Autodesk Inventor part; units mm, degrees
ref_plane "YZ Plane" through (0, 0, 0) normal (1, 0, 0) x (0, 1, 0)
ref_plane "XZ Plane" through (0, 0, 0) normal (0, 1, 0) x (-1, 0, 0)
ref_plane "XY Plane" through (0, 0, 0) normal (0, 0, 1) x (1, 0, 0)
sketch "草圖1" plane through (0, 0, 0) normal (0, 0, 1) x (1, 0, 0)
  line L0 (0, 0) -> (0, -20)
  line L1 (0, -20) -> (-115, -20)
  line L2 (0, -20) -> (450, -20)
  line L3 (167.5, 0) -> (430, 0)
  line L4 (167.5, 0) -> (-95, 0)
  line L5 (167.5, 75) -> (470, 75)
  line L6 (470, 75) -> (430, 0)
  line L7 (167.5, 75) -> (-135, 75)
  line L8 (-135, 75) -> (-95, 0)
  line L9 (130, 0) -> (130, 75)
  line L10 (130, 0) -> (150, 0)
  line L11 (150, 0) -> (150, 75)
  line L12 (167.5, 95) -> (545, 95)
  line L13 (545, 95) -> (545, 75)
  line L14 (545, 75) -> (500, 75)
  line L15 (500, 75) -> (450, -20)
  line L16 (-115, -20) -> (-165.6667, 75)
  line L17 (-165.6667, 75) -> (-210.6667, 75)
  line L18 (-210.6667, 75) -> (-210.6667, 95)
  line L19 (-210.6667, 95) -> (167.5, 95)
  dimension "d0" = 20
  dimension "d1" = 115
  dimension "d2" = 450
  dimension "d6" = 262.5
  dimension "d7" = 262.5
  dimension "d8" = 302.5
  dimension "d9" = 302.5
  dimension "d11" = 20
  dimension "d12" = 75
  dimension "d14" = 377.5
  dimension "d15" = 20
  dimension "d16" = 45
  dimension "d17" = 45
  dimension "d18" = 20
extrude "擠出1" add sketch "草圖1" along normal blind 20 contours L1 L16 L17 L18 L19 L12 L13 L14 L15 L2 | L9 L7 L11 L4
sketch "草圖2" plane through (-210.6667, 95, 0) normal (0, 1, 0) x (1, 0, 0)
  line L0 (0, 0) -> (0, -20)
  circle A0 centre (0, -10) radius 32.5
  circle A1 centre (32.5, -10) radius 5
  line L1 (755.6667, 0) -> (755.6667, -20)
  circle A2 centre (755.6667, -10) radius 32.5
  circle A3 centre (723.1667, -10) radius 5
  point P0 (210.6667, 0)
  dimension "d21" = 65
  dimension "d23" = 65
  dimension "d22" = 10
  dimension "d24" = 10
extrude "擠出2" add sketch "草圖2" along normal blind 20 contours A0 A1 | A0 A1 | A3 A2 | A2 A3 picked at (30.8705, -10.9665) picked at (33.9711, -11.3119) picked at (724.8619, -10) picked at (721.5286, -10)
sketch "草圖3" plane through (512.5, 115, 10) normal (0, 1, 0) x (1, 0, 0)
  circle A0 centre (0, 0) radius 17.5
  point P0 (-512.5, 10)
  dimension "d27" = 35
extrude "擠出3" add sketch "草圖3" along normal blind 10
sketch "草圖4" plane through (-178.1667, 115, 10) normal (0, 1, 0) x (1, 0, 0)
  circle A0 centre (0, 0) radius 5
  circle A1 centre (0, 0) radius 17.5
  point P0 (178.1667, 10)
  dimension "d30" = 35
extrude "擠出4" add sketch "草圖4" along normal blind 10 contours A0 | A1
properties part number "DOF8"
Geometry: final body of the model. Coordinates: model frame, mm. A direction names the side the tool comes from. Round coordinates to 2 decimals unless told otherwise and drop trailing zeros. Write each loop counter-clockwise with the first axis right and the second up, starting at its lowest first coordinate (ties: lowest second). Pieces come first, ordered by that corner, then holes. Notation, with made-up numbers: (21.5, 77) -> (34.5, 77) arc R19 cw to (34.5, 109) -> close; hole circle Ø3 at (67, 0.25). An arc over 180 degrees is marked (long way). Return JSON: item names as keys, results as strings.
Q1. Mould query, pull axis Y, two halves, no side actions, for faces 5 (the flat face through (-210.667, 85, 10)), 6 (the flat face through (-188, 75, 10)), 7 (the flat face through (512, 125, 10)), 8 (the flat face through (516, 115, 14)). Classes: +Y half, -Y half, draft (parallel to the pull), parting line (faces both ways), or undercut.
From the geometry:
{"face 5": "draft", "face 6": "-Y half", "face 7": "+Y half", "face 8": "undercut"}
Q2. Section C-C on y = -8.5. Return the cut outline in (x, z).
From the geometry:
{"outline": "(-121.13, 0) -> (456.05, 0) -> (456.05, 20) -> (-121.13, 20) -> close"}
Q3. Section A-A on x = 37. Return the cut outline in (y, z).
From the geometry:
{"outline": "(-20, 0) -> (0, 0) -> (0, 20) -> (-20, 20) -> close; (75, 0) -> (95, 0) -> (95, 20) -> (75, 20) -> close"}
Q4. Section B-B on y = 53. Return the cut outline in (x, z), and give its area (3 significant figures).
From the geometry:
{"outline": "(-153.93, 0) -> (-123.27, 0) -> (-123.27, 20) -> (-153.93, 20) -> close; (130, 0) -> (150, 0) -> (150, 20) -> (130, 20) -> close; (458.27, 0) -> (488.42, 0) -> (488.42, 20) -> (458.27, 20) -> close", "area": "1,620 mm2"}
Q5. Ray query, line 1 (Y direction, x = 279, z = 11.5); line 2 (Y direction, x = -114.5, z = 2.5); line 3 (Z direction, x = 270.5, y = -4.5). Return the intervals inside material, ascending.
From the geometry:
{"line 1": "-20 to 0, 75 to 95", "line 2": "-20 to 36.56, 75 to 95", "line 3": "0 to 20"}
Q6. First-contact query: pin 1 Ø16 at (y, z) = (51, 5.5) entering from -X; pin 2 Ø6 at (x, z) = (33, 14.5) entering from +Y; pin 3 Ø2 at (y, z) = (27.5, -0.5) entering from +X. Flat tips, straight axial feed; report the tip coordinate or a pass-through.
From the geometry:
{"pin 1": "x = -157.13", "pin 2": "y = 95", "pin 3": "x = 475.46"}
Q7. Set-up query: faces 1 (the flat face through (-174.52, 115, 13.64)), 2 (the flat face through (-115.28, 38.025, 9.86)), 3 (the cylindrical face through (-195.65, 119.93, 10.77)), 4 (the flat face through (-139.98, 26.84, 9.86)). Return all of +Z, -Z, +X, -X, +Y, -Y with unobstructed straight access to the full face (end or side cutting, diameter ignored); none if empty.
From the geometry:
{"face 1": "none", "face 2": "+Z, -Z", "face 3": "+Y", "face 4": "+Z, -Z, -X, -Y"}
